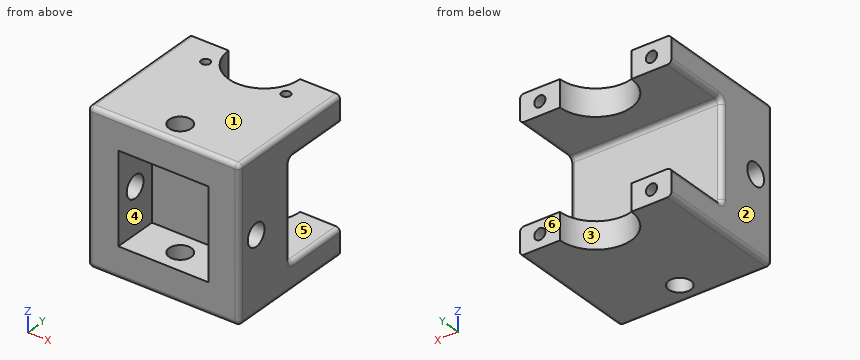
from build123d import *

# Parameters (mm, degrees)
SKETCH1_W           = 34
SKETCH1_H           = 34
BOSS_EXTRUDE1_DEPTH = 15
SKETCH2_W           = 20.2
SKETCH2_H           = 20.2
CUT_EXTRUDE1_DEPTH  = 10
SKETCH4_W           = 34
SKETCH4_H           = 15
BOSS_EXTRUDE2_DEPTH = 6
SKETCH7_R           = 8
CUT_EXTRUDE4_DEPTH  = 49.425200051
SKETCH17_R          = 1.25
CUT_EXTRUDE10_DEPTH = 10
SKETCH15_R          = 2.5
CUT_EXTRUDE8_DEPTH  = 49.425200051
SKETCH16_R          = 2.5
CUT_EXTRUDE9_DEPTH  = 49.425200051
FILLET2_R           = 1
SKETCH19_R          = 1
CUT_EXTRUDE12_DEPTH = 3


with BuildPart() as part:
    # Sketch1 → Boss-Extrude1 (new body)
    with BuildSketch(Plane(origin=(0, 0, 0), x_dir=(1, 0, 0), z_dir=(0, 1, 0))):
        Rectangle(SKETCH1_W, SKETCH1_H)
    extrude(amount=BOSS_EXTRUDE1_DEPTH)

    # Sketch2 → Cut-Extrude1 (cut)
    with BuildSketch(Plane.XZ):
        Rectangle(SKETCH2_W, SKETCH2_H)
    extrude(amount=-CUT_EXTRUDE1_DEPTH, mode=Mode.SUBTRACT)

    # Sketch4 → Boss-Extrude2 (add)
    with BuildSketch(Plane.XY.offset(17)):
        with Locations((0, 22.5)):
            Rectangle(SKETCH4_W, SKETCH4_H)
    boss_extrude2 = extrude(amount=-BOSS_EXTRUDE2_DEPTH)

    # Sketch7 → Cut-Extrude4 (cut, through all)
    with BuildSketch(Plane.XY.offset(17)):
        with Locations((0, 30)):
            Circle(SKETCH7_R)
    cut_extrude4 = extrude(amount=-CUT_EXTRUDE4_DEPTH, mode=Mode.SUBTRACT)

    # Sketch17 → Cut-Extrude10 (cut)
    with BuildSketch(Plane(origin=(0, 30, 0), x_dir=(1, 0, 0), z_dir=(0, 1, 0))):
        with Locations(Location((-12.5, -14, 0), (0, 0, 180))):
            Circle(SKETCH17_R)
        with Locations(Location((12.5, -14, 0), (0, 0, 180))):
            Circle(SKETCH17_R)
    cut_extrude10 = extrude(amount=-CUT_EXTRUDE10_DEPTH, mode=Mode.SUBTRACT)

    # Mirror1: Boss-Extrude2, Cut-Extrude4, Cut-Extrude10 across plane
    add(boss_extrude2.mirror(Plane.XY))
    add(cut_extrude4.mirror(Plane.XY), mode=Mode.SUBTRACT)
    add(cut_extrude10.mirror(Plane.XY), mode=Mode.SUBTRACT)

    # Sketch15 → Cut-Extrude8 (cut, through all)
    with BuildSketch(Plane(origin=(0, 0, -17), x_dir=(-1, 0, 0), z_dir=(0, 0, -1))):
        with Locations((0, 5)):
            Circle(SKETCH15_R)
    extrude(amount=-CUT_EXTRUDE8_DEPTH, mode=Mode.SUBTRACT)

    # Sketch16 → Cut-Extrude9 (cut, through all)
    with BuildSketch(Plane(origin=(17, 0, 0), x_dir=(0, 0, -1), z_dir=(1, 0, 0))):
        with Locations((0, 5)):
            Circle(SKETCH16_R)
    extrude(amount=-CUT_EXTRUDE9_DEPTH, mode=Mode.SUBTRACT)

    # Fillet2
    fillet2_edges = [part.edges().sort_by_distance(p)[0] for p in [
        (17, 15, 0),
        (17, 22.5, 11),
        (0, 15, 11),
        (-17, 22.5, 11),
        (0, 0, 17),
        (-17, 0, 0),
        (0, 0, -17),
        (17, 0, 0),
        (-17, 15, 0),
        (-17, 22.5, -11),
        (0, 15, -11),
        (17, 22.5, -11),
        (17, 15, 17),
        (-17, 15, 17),
        (-17, 15, -17),
        (17, 15, -17),
    ]]
    fillet(fillet2_edges, radius=FILLET2_R)

    # Sketch19 → Cut-Extrude12 (cut)
    with BuildSketch(Plane.XY.offset(17)):
        with Locations((-9, 24.5)):
            Circle(SKETCH19_R)
    cut_extrude12 = extrude(amount=-CUT_EXTRUDE12_DEPTH, mode=Mode.SUBTRACT)

    # Mirror2: Cut-Extrude12 across plane
    add(cut_extrude12.mirror(Plane(origin=(0, 0, 0), x_dir=(0, 0, 1), z_dir=(1, 0, 0))), mode=Mode.SUBTRACT)


solid = part.part
Input: part model. Units: mm. Frame: model coordinates. Face numbers are marked on the shaded views. A direction names the side the tool comes from. Give positions to 0.01 mm unless a question says otherwise; leave off trailing zeros. Loops run counter-clockwise (first coordinate to the right, second up) from the corner with the lowest first, then second, coordinate; pieces in that order, holes last. Notation, with made-up numbers: M 48.25,-3.5 L 105.25,-3.5 A13 cw 105.25,13.5 Z; hole C -3,20.5 d1. An arc over 180 degrees is marked long. Use CSV: the item, a comma, the result in double quotes.
(1) Set-up query: the marked faces 4, 5 and 6. Return all of +Z, -Z, +X, -X, +Y, -Y with unobstructed straight access to the full face (end or side cutting, diameter ignored); none if empty.
Outcome:
face 4,"-Y"
face 5,"+X, -X, +Y"
face 6,"+Z, -Z, +X, -X, +Y"
(2) Section C-C, the plane z = -14. Return loops of the section in (x, y).
Outcome:
outline,"M -17,1 A1 ccw -16,0 L 16,0 A1 ccw 17,1 L 17,30 L 13.75,30 L 13.75,20 L 11.25,20 L 11.25,30 L 8,30 A8 cw -8,30 L -11.25,30 L -11.25,20 L -13.75,20 L -13.75,30 L -17,30 Z; hole C 0,5 d5"
(3) Section D-D, the plane x = -12.5. Return loops of the section in (y, z), plus the area to 3 significant figures.
Outcome:
outline,"M 0,-16 A1 ccw 1,-17 L 30,-17 L 30,-15.25 L 20,-15.25 L 20,-12.75 L 30,-12.75 L 30,-11 L 16,-11 A1 cw 15,-10 L 15,10 A1 cw 16,11 L 30,11 L 30,12.75 L 20,12.75 L 20,15.25 L 30,15.25 L 30,17 L 1,17 A1 ccw 0,16 Z; hole C 5,0 d5"
area,"620 mm²"
(4) Section A-A, the plane y = 5. Return loops of the section in (x, z).
Outcome:
outline,"M -17,-16 A1 ccw -16,-17 L -2.5,-17 L -2.5,-10.1 L -10.1,-10.1 L -10.1,-2.5 L -17,-2.5 Z; M -17,2.5 L -10.1,2.5 L -10.1,10.1 L -2.5,10.1 L -2.5,17 L -16,17 A1 ccw -17,16 Z; M 2.5,-17 L 16,-17 A1 ccw 17,-16 L 17,-2.5 L 10.1,-2.5 L 10.1,-10.1 L 2.5,-10.1 Z; M 2.5,10.1 L 10.1,10.1 L 10.1,2.5 L 17,2.5 L 17,16 A1 ccw 16,17 L 2.5,17 Z"
(5) Pin query (flat end, axial travel): P1, Ø1, axis at x = 10.5, z = 2, coming from the +Y side; P2, Ø0.8, axis at x = 12.5, z = -14.5, coming from the +Y side; P3, Ø10, axis at x = 1, z = 1.5, coming from the -Y side. Return the tip coordinate at first contact, or that it passes through.
Outcome:
P1,"stops at y = 15"
P2,"stops at y = 20"
P3,"stops at y = 10"
(6) Pull-direction query (X, two-part tool) for the marked faces 1, 2 and 3; classes: pulls with the +X half, pulls with the -X half, needs draft (parallel to the pull), parting line crosses it, or undercut.
Outcome:
face 1,"needs draft"
face 2,"pulls with the -X half"
face 3,"undercut"
(7) Material intervals for L1, parallel to Z at x = 12.5, y = 23.5; L2, parallel to Z at x = 7, y = 25.5; L3, parallel to Y at x = -13.75, z = 0, sorted ascending. Write a range as [from, to].
Outcome:
L1,"z = [-17, -15.25], [-12.75, -11], [11, 12.75], [15.25, 17]"
L2,"z = [-17, -11], [11, 17]"
L3,"y = [0, 2.5], [7.5, 15]"
(8) Section B-B, the plane x = 0. Return loops of the section in (y, z).
Outcome:
outline,"M 0,-16 A1 ccw 1,-17 L 2.5,-17 L 2.5,-10.1 L 0,-10.1 Z; M 0,10.1 L 2.5,10.1 L 2.5,17 L 1,17 A1 ccw 0,16 Z; M 7.5,-17 L 22,-17 L 22,-11 L 16,-11 A1 cw 15,-10 L 15,10 A1 cw 16,11 L 22,11 L 22,17 L 7.5,17 L 7.5,10.1 L 10,10.1 L 10,-10.1 L 7.5,-10.1 Z"
